Work out the finished part from the listing and answer in its coordinate system (mm). Coordinates: 2 decimals unless noted, no trailing zeros. Order: outer loops, then holes, each group sorted by start corner. A loop starts at its lowest first (then second) coordinate and runs counter-clockwise, first axis right, second up.
1. The part is cut by section A-A, the plane x = 0. Count the separate pieces of the cut face and the enclosed holes in it, then the cut area to 3 significant figures.
2. The part is cut by section C-C, the plane y = 1. Give the vertices of the cut face in (x, z), then the cut area to 3 significant figures.
3. The part is cut by section D-D, the plane z = 5. Give the vertices of the cut face in (x, y), then the cut area to 3 significant figures.
4. Find the intervals of material crossed by probe 1 along X at (y, z) = (-0.75, 37); probe 2 along Z at (x, y) = (0, -3.35), in increasing order.
5. The part is cut by section B-B, the plane z = 74. Give the vertices of the cut face in (x, y).
6. A flat-ended cylindrical pin translates along its axis: pin 1 Ø4 at (x, z) = (0, 5) entering from +Y. Find the tip coordinate at first contact, or state that the pin passes through.
```python
from build123d import *

# Parameters (mm, degrees)
SKETCH_1_W          = 9
SKETCH_1_H          = 9
SKETCH_1_W_2        = 6
SKETCH_1_H_2        = 6
EXTRUDE_1_DEPTH     = 130
SKETCH_2_R          = 2.5
CUT_EXTRUDE_1_DEPTH = 90


with BuildPart() as part:
    # ｽｹｯﾁ1 → ﾎﾞｽ - 押し出し1 (new body)
    with BuildSketch(Plane.XY):
        Rectangle(SKETCH_1_W, SKETCH_1_H)
        Rectangle(SKETCH_1_W_2, SKETCH_1_H_2, mode=Mode.SUBTRACT)
    extrude(amount=EXTRUDE_1_DEPTH)

    # ｽｹｯﾁ2 → ｶｯﾄ - 押し出し1 (cut)
    with BuildSketch(Plane(origin=(0, 4.5, 0), x_dir=(1, 0, 0), z_dir=(0, 1, 0))):
        with Locations((0, -65)):
            Circle(SKETCH_2_R)
        with Locations((0, -5)):
            Circle(SKETCH_2_R)
        with Locations((0, -125)):
            Circle(SKETCH_2_R)
    extrude(amount=-CUT_EXTRUDE_1_DEPTH, mode=Mode.SUBTRACT)


solid = part.part
```
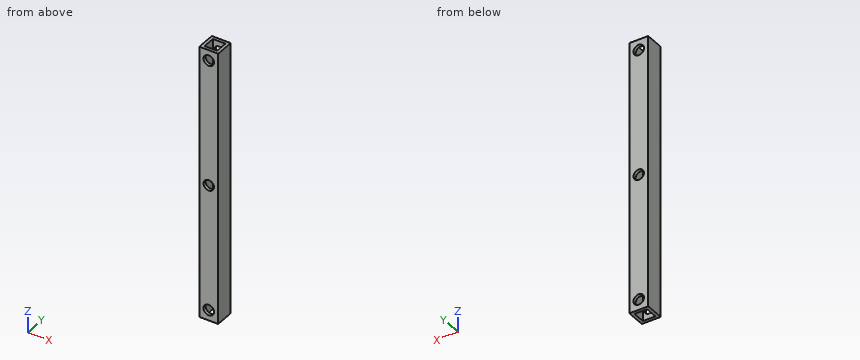
Geometry says:
1. separate pieces: 8
1. enclosed holes: 0
1. area: 345 mm2
2. outline: (-4.5, 0) - (-3, 0) - (-3, 130) - (-4.5, 130) - close; (3, 0) - (4.5, 0) - (4.5, 130) - (3, 130) - close
2. area: 390 mm2
3. outline: (-4.5, -4.5) - (-2.5, -4.5) - (-2.5, -3) - (-3, -3) - (-3, 3) - (-2.5, 3) - (-2.5, 4.5) - (-4.5, 4.5) - close; (2.5, -4.5) - (4.5, -4.5) - (4.5, 4.5) - (2.5, 4.5) - (2.5, 3) - (3, 3) - (3, -3) - (2.5, -3) - close
3. area: 30.0 mm2
4. probe 1: x = -4.5 to -3, 3 to 4.5
4. probe 2: z = 0 to 2.5, 7.5 to 62.5, 67.5 to 122.5, 127.5 to 130
5. outline: (-4.5, -4.5) - (4.5, -4.5) - (4.5, 4.5) - (-4.5, 4.5) - close; hole (-3, -3) - (3, -3) - (3, 3) - (-3, 3) - close
6. pin 1: passes through
